```python
from build123d import *

# Parameters (mm, degrees)
SKETCH1_W            = 143.4
SKETCH1_H            = 101.4
BOSS_EXTRUDE1_DEPTH  = 10
SKETCH2_W            = 121.8
SKETCH2_H            = 85.8
CUT_EXTRUDE1_DEPTH   = 89.382011744
CUT_EXTRUDE2_DEPTH   = 89.382011744
SKETCH4_W            = 2.25
SKETCH4_H            = 15
SKETCH4_W_2          = 15
SKETCH4_H_2          = 2.25
BOSS_EXTRUDE2_DEPTH  = 21.3
SKETCH5_W            = 6
SKETCH5_H            = 5
CUT_EXTRUDE3_DEPTH   = 107.925534836
SKETCH6_W            = 6
SKETCH6_H            = 5
CUT_EXTRUDE4_DEPTH   = 127.002142839
M3_CLEARANCE_HOLE1_D = 3.4
SKETCH10_W           = 12.5
SKETCH10_H           = 5
CUT_EXTRUDE5_DEPTH   = 127.002142839
CUT_EXTRUDE6_REACH   = 128.002
SKETCH11_W           = 12.5
SKETCH11_H           = 5
FILLET1_R            = 2.5
FILLET2_R            = 0.5
FILLET3_R            = 1
FILLET4_R            = 0.5


with BuildPart() as part:
    # Sketch1 → Boss-Extrude1 (new body)
    with BuildSketch(Plane(origin=(0, 0, 0), x_dir=(1, 0, 0), z_dir=(0, 1, 0))):
        Rectangle(SKETCH1_W, SKETCH1_H)
    extrude(amount=BOSS_EXTRUDE1_DEPTH)

    # Sketch2 → Cut-Extrude1 (cut, through all)
    with BuildSketch(Plane.XZ):
        Rectangle(SKETCH2_W, SKETCH2_H)
    extrude(amount=-CUT_EXTRUDE1_DEPTH, mode=Mode.SUBTRACT)

    # Sketch3 → Cut-Extrude2 (cut, through all)
    with BuildSketch(Plane.XZ):
        Polygon((-20, 50.7), (-20, 42.9), (-60.9, 42.9), (-60.9, -42.9), (20, -42.9), (20, -50.7), (-71.7, -50.7), (-71.7, 50.7), align=None)
    extrude(amount=-CUT_EXTRUDE2_DEPTH, mode=Mode.SUBTRACT)

    # Sketch4 → Boss-Extrude2 (add)
    with BuildSketch(Plane.XZ):
        with Locations((70.575, 0)):
            Rectangle(SKETCH4_W, SKETCH4_H)
        with Locations((0, 49.575)):
            Rectangle(SKETCH4_W_2, SKETCH4_H_2)
    extrude(amount=BOSS_EXTRUDE2_DEPTH)

    # Sketch5 → Cut-Extrude3 (cut, through all)
    with BuildSketch(Plane(origin=(71.7, 0, 0), x_dir=(0, 0, -1), z_dir=(1, 0, 0))):
        with Locations((0, -15.8)):
            Rectangle(SKETCH5_W, SKETCH5_H)
    extrude(amount=-CUT_EXTRUDE3_DEPTH, mode=Mode.SUBTRACT)

    # Sketch6 → Cut-Extrude4 (cut, through all)
    with BuildSketch(Plane.XY.offset(50.7)):
        with Locations((0, -15.8)):
            Rectangle(SKETCH6_W, SKETCH6_H)
    extrude(amount=-CUT_EXTRUDE4_DEPTH, mode=Mode.SUBTRACT)

    # M3 Clearance Hole1 (through all)
    with Locations(Plane(origin=(0, 10, 0), x_dir=(1, 0, 0), z_dir=(0, 1, 0))):
        with Locations((-15, -46.8), (25, 46.8)):
            Hole(M3_CLEARANCE_HOLE1_D / 2)

    # Sketch10 → Cut-Extrude5 (cut, through all)
    with BuildSketch(Plane.XY.offset(50.7)):
        with Locations((-13.75, 2.5)):
            Rectangle(SKETCH10_W, SKETCH10_H)
    extrude(amount=-CUT_EXTRUDE5_DEPTH, mode=Mode.SUBTRACT)

    # Sketch11 → Cut-Extrude6 (cut, up to next)
    with BuildSketch(Plane(origin=(0, 0, -50.7), x_dir=(-1, 0, 0), z_dir=(0, 0, -1)), mode=Mode.PRIVATE) as cut_extrude6_sk1:
        with Locations((-26.25, 7.5)):
            Rectangle(SKETCH11_W, SKETCH11_H)
    cut_extrude6_tool1 = extrude(cut_extrude6_sk1.sketch, amount=-CUT_EXTRUDE6_REACH, mode=Mode.PRIVATE) & part.part
    add(cut_extrude6_tool1.solids().sort_by_distance((26.25, 7.5, -50.7))[0], mode=Mode.SUBTRACT)

    # Fillet1
    fillet1_edges = [part.edges().sort_by_distance(p)[0] for p in [
        (71.7, 5, -50.7),
        (71.7, 5, 50.7),
    ]]
    fillet(fillet1_edges, radius=FILLET1_R)

    # Fillet2
    fillet2_edges = [part.edges().sort_by_distance(p)[0] for p in [
        (-7.5, 5, 46.8),
        (-20, 5, 46.8),
        (32.5, 10, -46.8),
        (32.5, 5, -46.8),
        (20, 5, -46.8),
        (-20, 10, 46.8),
        (20, 0, -46.8),
    ]]
    fillet(fillet2_edges, radius=FILLET2_R)

    # Fillet3
    fillet3_edges = [part.edges().sort_by_distance(p)[0] for p in [
        (69.45, 0, 0),
        (0, 0, 48.45),
    ]]
    fillet(fillet3_edges, radius=FILLET3_R)

    # Fillet4
    fillet4_edges = [part.edges().sort_by_distance(p)[0] for p in [
        (3, -13.3, 49.575),
        (3, -18.3, 49.575),
        (-3, -18.3, 49.575),
        (-3, -13.3, 49.575),
        (70.575, -13.3, -3),
        (70.575, -18.3, -3),
        (70.575, -18.3, 3),
        (70.575, -13.3, 3),
    ]]
    fillet(fillet4_edges, radius=FILLET4_R)


solid = part.part
```
Model file for the job. Use its own axes, mm. A direction names the side the tool comes from. Round coordinates to 2 decimals unless told otherwise and drop trailing zeros. Loops run counter-clockwise (first coordinate to the right, second up) from the corner with the lowest first, then second, coordinate; pieces in that order, holes last. Notation, with made-up numbers: M 24,77 L 35,77 A14 cw 35,86 Z; hole C -9.5,27 d10. An arc over 180 degrees is marked long. Put each result on its own line as item: value. Start each with the question number.
Item 1: Cut at D-D (x = 29). List the corners of the cut face in (y, z).
Item 2: Drop flat-ended pins along their axis: P1, Ø2.5, axis at x = -15, z = 46.8, coming from the -Y side; P2, Ø4, axis at x = 27, z = -47.5, coming from the +Y side; P3, Ø11, axis at y = 7, z = 7.5, coming from the -X side; P4, Ø1.6, axis at y = -10.5, z = 49.5, coming from the +X side. Give the stop position or say it passes through.
Item 3: Cut at C-C (z = -46.8). List the corners of the cut face in (x, y).
Item 4: Cut at B-B (x = 41.5). List the corners of the cut face in (y, z), then the cut area to 3 significant figures.
Item 5: Drill centre lines: line 1 along Z through (x, y) = (25, 2.6); line 2 along X through (y, z) = (8.8, 46.8); line 3 along Z through (x, y) = (-15, 8.9). Where is each one in solid material? Low to high.
Item 6: Cut at A-A (y = -16). List the corners of the cut face in (x, z), then the cut area to 3 significant figures.
Item 7: 3-axis set-ups, long thin cutter, end or side, ignore diameter. For faces 5 (the face through (60.9, 5, -1)), 6 (the face through (71, -16, 3)), 7 (the face through (3, -16, 50)): which of +Z, -Z, +X, -X, +Y, -Y reach the whole face in a straight line?
Item 8: Mould opens along Y. For faces 1 (the face through (71, -18.3, 0)), 2 (the face through (14, 1, 50.7)), 3 (the face through (63, 10, 11)), 4 (the face through (0, -21.3, 50)) say: released by +Y, released by -Y, zero draft, split by the parting line, or undercut.
Answer block:
1. outline: M 0,-50.7 L 5,-50.7 L 5,-42.9 L 0,-42.9 Z; M 0,42.9 L 10,42.9 L 10,50.7 L 0,50.7 Z
2. P1: through
2. P2: y = 5
2. P3: x = 60.9
2. P4: x = 7.5
3. outline: M 20,0.5 A0.5 ccw 20.5,0 L 23.3,0 L 23.3,5 L 20.5,5 A0.5 ccw 20,4.5 Z; M 26.7,0 L 71.7,0 L 71.7,10 L 33,10 A0.5 ccw 32.5,9.5 L 32.5,5.5 A0.5 cw 32,5 L 26.7,5 Z
4. outline: M 0,-50.7 L 10,-50.7 L 10,-42.9 L 0,-42.9 Z; M 0,42.9 L 10,42.9 L 10,50.7 L 0,50.7 Z
4. area: 156 mm2
5. line 1: -50.7 to -48.5, -45.1 to -42.9, 42.9 to 50.7
5. line 2: -20 to -16.7, -13.3 to 71.7
5. line 3: 42.9 to 45.1, 48.5 to 50.7
6. outline: M -7.5,48.45 L -3,48.45 L -3,50.7 L -7.5,50.7 Z; M 3,48.45 L 7.5,48.45 L 7.5,50.7 L 3,50.7 Z; M 69.45,-7.5 L 71.7,-7.5 L 71.7,-3 L 69.45,-3 Z; M 69.45,3 L 71.7,3 L 71.7,7.5 L 69.45,7.5 Z
6. area: 40.5 mm2
7. face 5: -X, +Y, -Y
7. face 6: +X, -X
7. face 7: +Z, -Z
8. face 1: undercut
8. face 2: zero draft
8. face 3: released by +Y
8. face 4: released by -Y
